Verification items for this drawing (mm, ordinates from the low corner). A direction names the side the tool comes from. Round coordinates to 2 decimals unless told otherwise and drop trailing zeros. Loops run counter-clockwise (first coordinate to the right, second up) from the corner with the lowest first, then second, coordinate; pieces in that order, holes last. Notation, with made-up numbers: M -6.75,82 L 34.25,82 A24 cw 34.25,106 Z; hole C 24.25,-38.75 d11. An arc over 180 degrees is marked long. Answer in a Markdown table with one row per item. Add a question column.
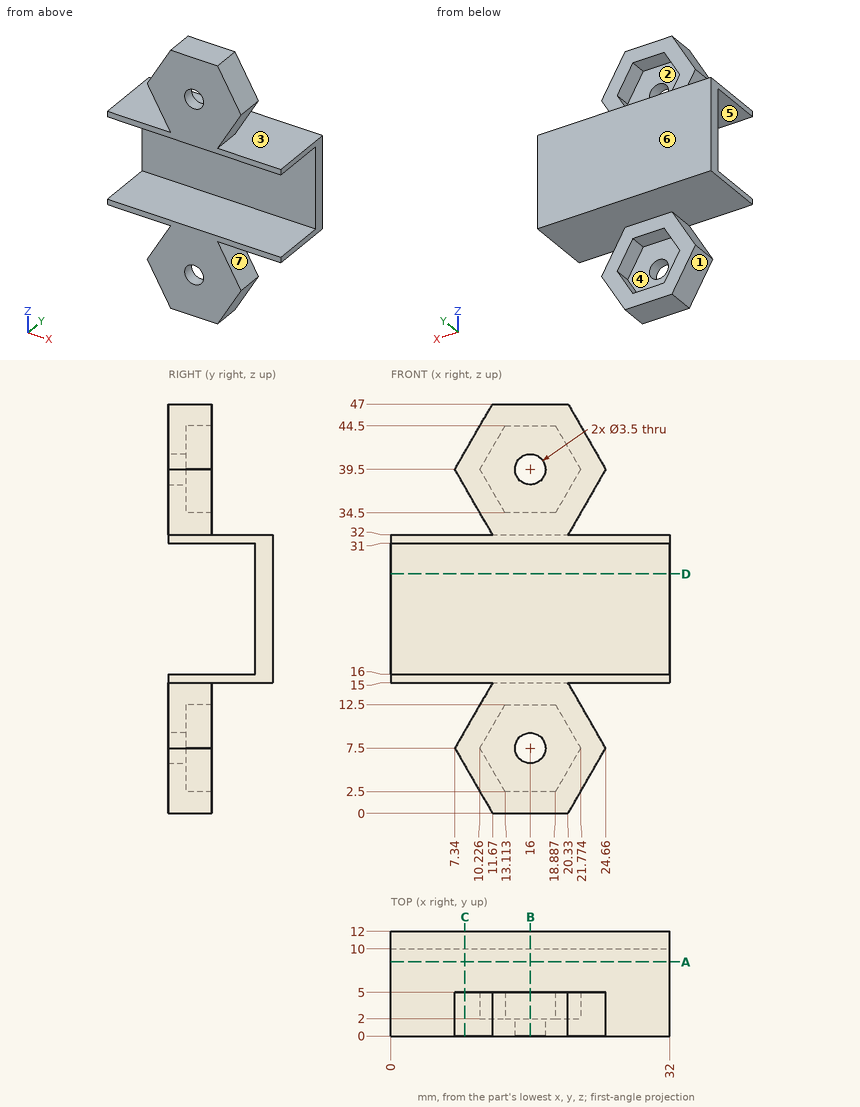
1) Cross-section at A-A, the plane y = 8.5. Record the boundary of the cut face in (x, z).
2) Cross-section at D-D, the plane z = 27.5. Record the boundary of the cut face in (x, y).
3) Cross-section at C-C, the plane x = 8.5. Record the boundary of the cut face in (y, z).
4) Draft check along X on the marked faces 1, 2 and 3. Enter one of: +X half, -X half, draft (parallel to the pull), parting line (faces both ways), or undercut.
5) Thickness scan on L1, parallel to Z at x = 30, y = 5.5; L2, parallel to Z at x = 18.5, y = 3.25; L3, parallel to Z at x = 13, y = 3.75 (1 decimal). Record the ranges inside material, lowest first. Write a range as [from, to].
6) Cross-section at B-B, the plane x = 16. Record the boundary of the cut face in (y, z).
7) Set-up check for the marked faces 4, 5, 6 and 7: record each of +Z, -Z, +X, -X, +Y, -Y from which the full face is reachable in a straight line by a thin tool's end or side.
8) Go/stop test with flat-tipped pins: pin 1 (3 mm diameter, centred on x = 26, z = 9.5, fed in from -Y); pin 2 (7.5 mm diameter, centred on x = 15, z = 42.5, fed in from +Y); pin 3 (7.5 mm diameter, centred on x = 21, z = 21, fed in from -Y); pin 4 (3 mm diameter, centred on x = 13.5, z = 7, fed in from +Y). Record where each tip stops, or that it passes through.
Worked answers:
| question | item | result |
|---|---|---|
| 1 | outline | M 0,15 L 32,15 L 32,16 L 0,16 Z; M 0,31 L 32,31 L 32,32 L 0,32 Z |
| 2 | outline | M 0,10 L 32,10 L 32,12 L 0,12 Z |
| 3 | outline | M 0,5.49 L 5,5.49 L 5,9.51 L 0,9.51 Z; M 0,15 L 12,15 L 12,32 L 0,32 L 0,31 L 10,31 L 10,16 L 0,16 Z; M 0,37.49 L 5,37.49 L 5,41.51 L 0,41.51 Z |
| 4 | face 1 | -X half |
| 4 | face 2 | undercut |
| 4 | face 3 | draft |
| 5 | L1 | z = [15, 16], [31, 32] |
| 5 | L2 | z = [0, 2.5], [12.5, 16], [31, 34.5], [44.5, 47] |
| 5 | L3 | z = [0, 2.7], [12.3, 16], [31, 34.7], [44.3, 47] |
| 6 | outline | M 0,0 L 5,0 L 5,2.5 L 2,2.5 L 2,5.75 L 0,5.75 Z; M 0,9.25 L 2,9.25 L 2,12.5 L 5,12.5 L 5,15 L 12,15 L 12,32 L 5,32 L 5,34.5 L 2,34.5 L 2,37.75 L 0,37.75 L 0,31 L 10,31 L 10,16 L 0,16 Z; M 0,41.25 L 2,41.25 L 2,44.5 L 5,44.5 L 5,47 L 0,47 Z |
| 7 | face 4 | +Y |
| 7 | face 5 | +X, -X, -Y |
| 7 | face 6 | +Z, -Z, +X, -X, +Y |
| 7 | face 7 | +X, +Y, -Y |
| 8 | pin 1 | passes through |
| 8 | pin 2 | stops at y = 5 |
| 8 | pin 3 | stops at y = 10 |
| 8 | pin 4 | stops at y = 2 |
